The listing builds one solid part. Answer for the finished solid, in the listing's coordinates (mm). Face numbers are marked on the shaded views. A direction names the side the tool comes from. Give positions to 0.01 mm unless a question says otherwise; leave off trailing zeros. Loops run counter-clockwise (first coordinate to the right, second up) from the corner with the lowest first, then second, coordinate; pieces in that order, holes last. Notation, with made-up numbers: M 16,41 L 26,41 A19 ccw 26,53 Z; hole C 50,39.5 d1. An arc over 180 degrees is marked long. Return JSON: item names as keys, results as strings.
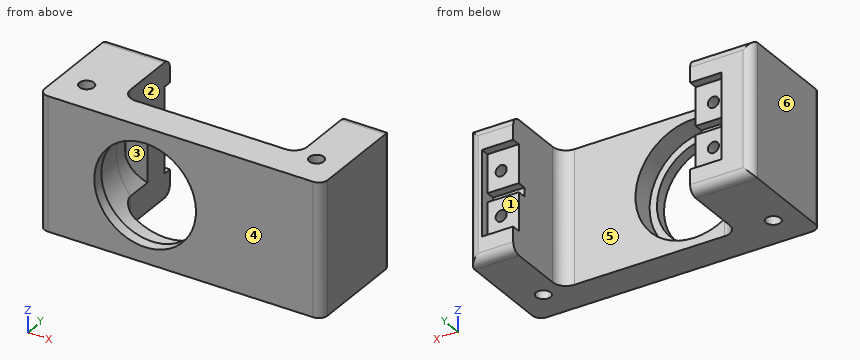
from build123d import *

# Parameters (mm, degrees)
SKETCH_1_W             = 64
SKETCH_1_H             = 30
EXTRUDE_555_DEPTH      = 7.5
SKETCH_2_R             = 13.175
CUT_EXTRUDE_693_DEPTH  = 5
SKETCH_4_R             = 11.5
CUT_EXTRUDE_912_DEPTH  = 44.011626335
EXTRUDE_START          = 3
SKETCH_8_W             = 64
SKETCH_8_H             = 30
SKETCH_8_R             = 13.175
EXTRUDE_1127_DEPTH     = 3
EXTRUDE_START_2        = 12
SKETCH_9_W             = 10
SKETCH_9_H             = 30
EXTRUDE_1452_DEPTH     = 12
SKETCH_10_R            = 1.25
CUT_EXTRUDE_1739_DEPTH = 11
SKETCH_11_R            = 1.65
CUT_EXTRUDE_2260_DEPTH = 55.829280499
SKETCH_12_W            = 10
SKETCH_12_H            = 5.4
EXTRUDE_2664_DEPTH     = 2
CUT_EXTRUDE_2902_DEPTH = 3
SKETCH_15_W            = 10
SKETCH_15_H            = 19.2
SKETCH_15_R            = 1.25
EXTRUDE_3173_DEPTH     = 9
CHAMFER_5_SIZE         = 3
SKETCH_17_W            = 2.9
SKETCH_17_H            = 19.2
EXTRUDE_3597_DEPTH     = 2
SKETCH_16_W            = 7.1
SKETCH_16_H            = 2
CUT_EXTRUDE_3878_DEPTH = 2
SKETCH_18_W            = 4
SKETCH_18_H            = 30
EXTRUDE_4043_DEPTH     = 14
FILLET_4_R             = 3
FILLET_5_R             = 2


with BuildPart() as part:
    # Эскиз1 → Extrude 555 (new body)
    with BuildSketch(Plane(origin=(0, 0, 0), x_dir=(1, 0, 0), z_dir=(0, 1, 0))):
        with Locations((8, 0)):
            Rectangle(SKETCH_1_W, SKETCH_1_H)
    extrude(amount=EXTRUDE_555_DEPTH)

    # Эскиз2 → Cut-Extrude 693 (cut)
    with BuildSketch(Plane(origin=(0, 7.5, 0), x_dir=(1, 0, 0), z_dir=(0, 1, 0))):
        with Locations(Location((0, 0, 0), (0, 0, 270))):
            Circle(SKETCH_2_R)
    extrude(amount=-CUT_EXTRUDE_693_DEPTH, mode=Mode.SUBTRACT)

    # Эскиз4 → Cut-Extrude 912 (cut, through all)
    with BuildSketch(Plane(origin=(0, 2.5, 0), x_dir=(1, 0, 0), z_dir=(0, 1, 0))):
        with Locations(Location((0, 0, 0), (0, 0, 270))):
            Circle(SKETCH_4_R)
    extrude(amount=-CUT_EXTRUDE_912_DEPTH, mode=Mode.SUBTRACT)

    # Эскиз8 → Extrude 1127 (add)
    with BuildSketch(Plane(origin=(0, 7.5, 0), x_dir=(1, 0, 0), z_dir=(0, 1, 0)).offset(EXTRUDE_START)):
        with Locations((8, 0)):
            Rectangle(SKETCH_8_W, SKETCH_8_H)
        with Locations(Location((0, 0, 0), (0, 0, 270))):
            Circle(SKETCH_8_R, mode=Mode.SUBTRACT)
    extrude(amount=-EXTRUDE_1127_DEPTH)

    # Эскиз9 → Extrude 1452 (add)
    with BuildSketch(Plane(origin=(0, 10.5, 0), x_dir=(1, 0, 0), z_dir=(0, 1, 0)).offset(EXTRUDE_START_2)):
        with BuildLine():
            Line((-20, 15), (-10, 15))
            Line((-10, 15), (-10, 8.577914956))
            ThreePointArc((-10, 8.577914956), (-13.175, 0), (-10, -8.577914956))
            Line((-10, -8.577914956), (-10, -15))
            Line((-10, -15), (-20, -15))
            Line((-20, -15), (-20, 15))
        make_face()
        with Locations((35, 0)):
            Rectangle(SKETCH_9_W, SKETCH_9_H)
    extrude(amount=-EXTRUDE_1452_DEPTH)

    # Эскиз10 → Cut-Extrude 1739 (cut)
    with BuildSketch(Plane(origin=(0, 22.5, 0), x_dir=(1, 0, 0), z_dir=(0, 1, 0))):
        with Locations(Location((-14, 5, 0), (0, 0, 270))):
            Circle(SKETCH_10_R)
        with Locations(Location((-14, -5, 0), (0, 0, 270))):
            Circle(SKETCH_10_R)
        with Locations(Location((34, -5, 0), (0, 0, 270))):
            Circle(SKETCH_10_R)
        with Locations(Location((34, 5, 0), (0, 0, 270))):
            Circle(SKETCH_10_R)
    extrude(amount=-CUT_EXTRUDE_1739_DEPTH, mode=Mode.SUBTRACT)

    # Эскиз11 → Cut-Extrude 2260 (cut, through all)
    with BuildSketch(Plane.XY.offset(15)):
        with Locations((-18, 7.5)):
            Circle(SKETCH_11_R)
        with Locations((34, 7.5)):
            Circle(SKETCH_11_R)
    extrude(amount=-CUT_EXTRUDE_2260_DEPTH, mode=Mode.SUBTRACT)

    # Эскиз12 → Extrude 2664 (add)
    with BuildSketch(Plane(origin=(0, 22.5, 0), x_dir=(1, 0, 0), z_dir=(0, 1, 0))):
        with Locations((-15, 12.3)):
            Rectangle(SKETCH_12_W, SKETCH_12_H)
        with Locations((-15, -12.3)):
            Rectangle(SKETCH_12_W, SKETCH_12_H)
        with Locations((35, -12.3)):
            Rectangle(SKETCH_12_W, SKETCH_12_H)
        with Locations((35, 12.3)):
            Rectangle(SKETCH_12_W, SKETCH_12_H)
    extrude(amount=EXTRUDE_2664_DEPTH)

    # Эскиз14 → Cut-Extrude 2902 (cut)
    with BuildSketch(Plane(origin=(0, 10.5, 0), x_dir=(1, 0, 0), z_dir=(0, 1, 0))):
        with BuildLine():
            Line((-10, 15), (-10, 8.577914956))
            ThreePointArc((-10, 8.577914956), (13.175, 0), (-10, -8.577914956))
            Line((-10, -8.577914956), (-10, -15))
            Line((-10, -15), (30, -15))
            Line((30, -15), (30, 15))
            Line((30, 15), (-10, 15))
        make_face()
    extrude(amount=-CUT_EXTRUDE_2902_DEPTH, mode=Mode.SUBTRACT)

    # Эскиз15 → Extrude 3173 (add)
    with BuildSketch(Plane(origin=(0, 22.5, 0), x_dir=(1, 0, 0), z_dir=(0, 1, 0))):
        with Locations((-15, 0)):
            Rectangle(SKETCH_15_W, SKETCH_15_H)
        with Locations(Location((-14, 5, 0), (0, 0, 270))):
            Circle(SKETCH_15_R, mode=Mode.SUBTRACT)
        with Locations(Location((-14, -5, 0), (0, 0, 270))):
            Circle(SKETCH_15_R, mode=Mode.SUBTRACT)
    extrude(amount=-EXTRUDE_3173_DEPTH)

    # Фаска5
    chamfer_5_edges = [part.edges().sort_by_distance(p)[0] for p in [
        (-10, 13.5, 0),
    ]]
    chamfer(chamfer_5_edges, length=CHAMFER_5_SIZE)

    # Эскиз17 → Extrude 3597 (add)
    with BuildSketch(Plane(origin=(0, 22.5, 0), x_dir=(1, 0, 0), z_dir=(0, 1, 0))):
        with Locations((-18.55, 0)):
            Rectangle(SKETCH_17_W, SKETCH_17_H)
        with Locations((38.55, 0)):
            Rectangle(SKETCH_17_W, SKETCH_17_H)
    extrude(amount=EXTRUDE_3597_DEPTH)

    # Эскиз16 → Cut-Extrude 3878 (cut)
    with BuildSketch(Plane(origin=(0, 22.5, 0), x_dir=(1, 0, 0), z_dir=(0, 1, 0))):
        with Locations((-13.55, 0)):
            Rectangle(SKETCH_16_W, SKETCH_16_H)
        with Locations((33.55, 0)):
            Rectangle(SKETCH_16_W, SKETCH_16_H)
    extrude(amount=-CUT_EXTRUDE_3878_DEPTH, mode=Mode.SUBTRACT)

    # Эскиз18 → Extrude 4043 (add)
    with BuildSketch(Plane(origin=(0, 10.5, 0), x_dir=(1, 0, 0), z_dir=(0, 1, 0))):
        with Locations((-22, 0)):
            Rectangle(SKETCH_18_W, SKETCH_18_H)
    extrude(amount=EXTRUDE_4043_DEPTH)

    # Скругление4
    fillet_4_edges = [part.edges().sort_by_distance(p)[0] for p in [
        (30, 7.5, 0),
        (-10, 7.5, 11.788957478),
        (-10, 7.5, -11.788957478),
    ]]
    fillet(fillet_4_edges, radius=FILLET_4_R)

    # Скругление5
    fillet_5_edges = [part.edges().sort_by_distance(p)[0] for p in [
        (-17, 24.5, 15),
        (40, 24.5, 0),
        (35, 24.5, 15),
        (35, 24.5, -15),
        (-24, 24.5, 0),
        (40, 0, 0),
        (-24, 0, 0),
        (-17, 24.5, -15),
    ]]
    fillet(fillet_5_edges, radius=FILLET_5_R)


solid = part.part
(1) The part is cut by section C-C (x = -18). Determine the outline of the cut face in (y, z), and give its area (3 significant figures).
Values follow:
{"outline": "M 0,-15 L 5.85,-15 L 5.85,15 L 0,15 Z; M 9.15,-15 L 22.5,-15 A2 ccw 24.5,-13 L 24.5,13 A2 ccw 22.5,15 L 9.15,15 Z", "area": "634 mm²"}
(2) Given pin 1 (12 mm diameter, centred on x = 10, z = 3.5, fed in from +Y); pin 2 (2 mm diameter, centred on x = 32.5, z = -6.5, fed in from +Y); pin 3 (1 mm diameter, centred on x = 34, y = 24, fed in from +Z); pin 4 (8 mm diameter, centred on x = 3, z = -5, fed in from +Y), each flat-ended and moving along its own axis, determine where each tip first touches the part or whether it passes through.
Values follow:
{"pin 1": "y = 7.5", "pin 2": "y = 22.5", "pin 3": "z = 14.73", "pin 4": "through"}
(3) Straight lines are drawn through the part: line 1 along X through (y, z) = (19.5, 5); line 2 along X through (y, z) = (15, 5); line 3 along X through (y, z) = (18.5, 6.5). For each, find the intervals that lie inside material, in ascending order.
Values follow:
{"line 1": "-24 to -15.25, -12.75 to -10, 30 to 32.75, 35.25 to 40", "line 2": "-24 to -15.25, -12.75 to -11.5, 30 to 32.75, 35.25 to 40", "line 3": "-24 to -10, 30 to 40"}
(4) The part is cut by section D-D (x = 34). Determine the outline of the cut face in (y, z), and give its area (3 significant figures).
Values follow:
{"outline": "M 0,-15 L 5.85,-15 L 5.85,15 L 0,15 Z; M 9.15,-15 L 22.5,-15 A2 ccw 24.5,-13 L 24.5,-9.6 L 22.5,-9.6 L 22.5,-6.25 L 11.5,-6.25 L 11.5,-3.75 L 22.5,-3.75 L 22.5,-1 L 20.5,-1 L 20.5,1 L 22.5,1 L 22.5,3.75 L 11.5,3.75 L 11.5,6.25 L 22.5,6.25 L 22.5,9.6 L 24.5,9.6 L 24.5,13 A2 ccw 22.5,15 L 9.15,15 Z", "area": "537 mm²"}
(5) The part is cut by section B-B (y = 19.5). Determine the outline of the cut face in (x, z).
Values follow:
{"outline": "M -24,-15 L -10,-15 L -10,15 L -24,15 Z; M 30,-15 L 40,-15 L 40,15 L 30,15 Z; hole C -14,-5 d2.5; hole C -14,5 d2.5; hole C 34,-5 d2.5; hole C 34,5 d2.5"}
(6) A tool of negligible diameter and unlimited length cuts with its end or side. For the marked faces 1, 2 and 3, from which of +Z, -Z, +X, -X, +Y, -Y can it reach the whole face along a straight path? Write none if from no direction.
Values follow:
{"face 1": "+Y", "face 2": "+Z, -Z, +Y", "face 3": "none"}
(7) Determine the mould class of the marked faces 4, 5 and 6 for opening direction X: released by +X, released by -X, zero draft, split by the parting line, or undercut.
Values follow:
{"face 4": "zero draft", "face 5": "undercut", "face 6": "released by -X"}
(8) The part is cut by section A-A (z = 0). Determine the outline of the cut face in (x, y) (3 decimals).
Values follow:
{"outline": "M -24,2 A2 ccw -22,0 L -11.5,0 L -11.5,2.5 L -13.175,2.5 L -13.175,13.5 L -13,13.5 L -10,16.5 L -10,20.5 L -17.1,20.5 L -17.1,24.5 L -22,24.5 A2 ccw -24,22.5 Z; M 11.5,0 L 38,0 A2 ccw 40,2 L 40,22.5 A2 ccw 38,24.5 L 37.1,24.5 L 37.1,20.5 L 30,20.5 L 30,10.5 A3 cw 27,7.5 L 13.175,7.5 L 13.175,2.5 L 11.5,2.5 Z; hole C -18,7.5 d3.3; hole C 34,7.5 d3.3"}
